Here's how the part is built. I have some questions about the finished solid (model axes, mm). Face numbers are marked on the shaded views. Coordinates: 2 decimals unless noted, no trailing zeros. Write each loop counter-clockwise with the first axis right and the second up, starting at its lowest first coordinate (ties: lowest second). Pieces come first, ordered by that corner, then holes. Notation, with made-up numbers: (-9.5, 1.25) - (35.5, 1.25) arc R24 ccw to (35.5, 30.25) - close; hole circle Ø9 at (-7, -32). An arc over 180 degrees is marked (long way). Answer in a Markdown table with one row per item. Add a question column.
Item 1: Imagine slicing it at C-C (x = -2.75). Please give me the cut outline in (y, z) (1 decimal).
Item 2: I'm going to push flat-ended pins straight in: pin 1 (3 mm diameter, centred on y = -1.5, z = -0.5, fed in from -X); pin 2 (1 mm diameter, centred on x = -3, y = 2.5, fed in from +Z); pin 3 (1.5 mm diameter, centred on y = -0.5, z = -1.5, fed in from +X); pin 4 (4 mm diameter, centred on x = -3.5, z = 2, fed in from +Y). Where does each tip first touch, or does it pass through?
Item 3: Imagine slicing it at A-A (y = 0). Please give me the cut outline in (x, z).
Item 4: We'd pull the mould along Y, two halves only. Please class the marked faces 1, 2 and 3: +Y half, -Y half, draft (parallel to the pull), parting line (faces both ways), or undercut.
Item 5: Imagine slicing it at B-B (x = -9.75). Please give me the cut outline in (y, z), plus the area to 3 significant figures.
Item 6: If I drill on probe 1 along Z at (x, y) = (-9.25, 0); probe 2 along Z at (x, y) = (-1.5, 2.5), over which ranges is the centre line in solid material (lowest first)? Write a range as from..to.
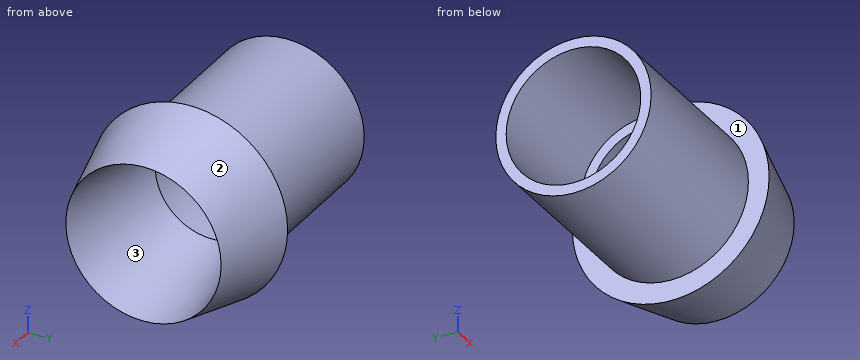
Autodesk Inventor part; units mm, degrees
ref_plane "YZ Plane" through (0, 0, 0) normal (1, 0, 0) x (0, 1, 0)
ref_plane "XZ Plane" through (0, 0, 0) normal (0, 1, 0) x (-1, 0, 0)
ref_plane "XY Plane" through (0, 0, 0) normal (0, 0, 1) x (1, 0, 0)
sketch "Эскиз1" plane through (0, 0, 0) normal (0, 0, 1) x (1, 0, 0)
  line L0 (0, 0) -> (-21.4884, 0)
  line L1 (0, 3.75) -> (-4, 4.75)
  line L2 (-4, 4.75) -> (-4, 3.75)
  line L3 (-4, 3.75) -> (-12.5, 3.75)
  line L4 (-12.5, 3.75) -> (-12.5, 3.25)
  line L5 (-12.5, 3.25) -> (-6, 3.25)
  line L6 (-6, 3.25) -> (-6, 2.75)
  line L7 (-6, 2.75) -> (0, 3.75)
  dimension "d1" = 8.5
  dimension "d2" = 1
  dimension "d3" = 0.5
  dimension "d4" = 6.5
  dimension "d5" = 4
  dimension "d6" = 0
  dimension "d9" = 3.75
  dimension "d10" = 2.75
  dimension "d11" = 3.75
revolve "Вращение1" add sketch "Эскиз1" angle 360 about axis through (0, 0, 0) along (-1, 0, 0)
properties part number "корпус фары"
Here are the results:
| question | item | result |
|---|---|---|
| 1 | outline | circle Ø8.9 at (0, 0); hole circle Ø6.6 at (0, 0) |
| 2 | pin 1 | stops at x = -6 |
| 2 | pin 2 | stops at z = 4.07 |
| 2 | pin 3 | passes through |
| 2 | pin 4 | stops at y = 4.75 |
| 3 | outline | (-12.5, -3.75) - (-4, -3.75) - (-4, -4.75) - (0, -3.75) - (-6, -2.75) - (-6, -3.25) - (-12.5, -3.25) - close; (-12.5, 3.25) - (-6, 3.25) - (-6, 2.75) - (0, 3.75) - (-4, 4.75) - (-4, 3.75) - (-12.5, 3.75) - close |
| 4 | face 1 | draft |
| 4 | face 2 | parting line |
| 4 | face 3 | undercut |
| 5 | outline | circle Ø7.5 at (0, 0); hole circle Ø6.5 at (0, 0) |
| 5 | area | 11.0 mm2 |
| 6 | probe 1 | z = -3.75..-3.25, 3.25..3.75 |
| 6 | probe 2 | z = -3.28..-2.45, 2.45..3.28 |
